Check sheet for the modelled part. Datum: model origin and axes. Units: mm. A direction names the side the tool comes from. Coordinates: 2 decimals unless noted, no trailing zeros. Loops run counter-clockwise (first coordinate to the right, second up) from the corner with the lowest first, then second, coordinate; pieces in that order, holes last. Notation, with made-up numbers: (77.25, 67.25) -> (125.25, 67.25) arc R29 ccw to (125.25, 87.25) -> close; hole circle Ø5 at (53.25, 51). An arc over 180 degrees is marked (long way). Use one line per item in the form item = value.
Autodesk Inventor part; units mm, degrees
ref_plane "YZ Plane" through (0, 0, 0) normal (1, 0, 0) x (0, 1, 0)
ref_plane "XZ Plane" through (0, 0, 0) normal (0, 1, 0) x (-1, 0, 0)
ref_plane "XY Plane" through (0, 0, 0) normal (0, 0, 1) x (1, 0, 0)
sketch "Sketch2" plane through (0, 0, 0) normal (0, 1, 0) x (-1, 0, 0)
  arc A0 (-315.9842, -7.0824) -> (-308.3642, -3.3824) centre (-312.1742, -5.2324) ccw
  line L0 (-312.1742, -5.2324) -> (-308.3642, -3.3824) construction
  line L1 (-312.1742, -5.2324) -> (-315.9842, -7.0824) construction
  line L2 (-343.9242, 64.6176) -> (-343.9242, 51.9176)
  line L3 (-343.9242, 64.6176) -> (-343.9242, 53.0352)
  line L4 (-343.9242, 64.6176) -> (-333.7642, 64.6176)
  arc A1 (-343.9242, 51.9176) -> (-343.2864, 49.1439) centre (-337.5742, 51.9176) ccw
  line L5 (-315.9842, -7.0824) -> (-343.2864, 49.1439)
  line L6 (-333.7642, 64.6176) -> (-333.7642, 50.3868)
  arc A2 (-333.7642, 50.3868) -> (-333.1264, 47.6131) centre (-327.4142, 50.3868) ccw
  line L7 (-333.1264, 47.6131) -> (-308.3642, -3.3824)
  circle A3 centre (-337.5742, 58.2676) radius 2.1463
  circle A4 centre (-312.1742, -5.2324) radius 2.1463
  circle A5 centre (-326.0427, 23.3285) radius 2.1463
  point P0 (0, 0)
  dimension "d0" = 180
  dimension "d1" = 3.81
  dimension "d2" = 10.16
  dimension "d3" = 12.7
  dimension "d4" = 6.35
  dimension "d5" = 31.75
  dimension "d6" = 69.85
  dimension "d7" = 6.35
  dimension "d8" = 4.2926
  dimension "d9" = 4.2926
  dimension "d10" = 6.35
  dimension "d11" = 6.35
  dimension "d12" = 4.2926
  dimension "d13" = 31.75
  dimension "d14" = 4.2354
extrude "Extrusion1" add sketch "Sketch2" along normal blind 1.5875
properties part number "Front Guard"
(1) Tool access check on faces 1 (the flat face through (333.764, 1, 58)), 2 (the flat face through (329, 0, 28)). Record the directions out of +Z, -Z, +X, -X, +Y, -Y that give a thin tool (end or side, any length) a straight path to the whole face; none if there is none.
Established:
face_1 = +Z, -X, +Y, -Y
face_2 = +Z, -Z, +X, -X, -Y
(2) Mould release check, pull along X, two halves, no side actions. Record for faces 3 (the cylindrical face through (339.72, 0.78, 58.17)), 4 (the cylindrical face through (310.24, 0.78, -9)), 5 (the flat face through (320.919, 0.783, 22.472)): +X half, -X half, draft (parallel to the pull), parting line (faces both ways), or undercut.
Established:
face_3 = undercut
face_4 = parting line
face_5 = -X half
(3) Go/stop test with flat-tipped pins: P1, Ø3.5, axis at x = 326.04, z = 23.33, coming from the +Y side; P2, Ø12, axis at x = 325, z = 19.5, coming from the -Y side. Record where each tip stops, or that it passes through.
Established:
P1 = through
P2 = 0
(4) Section check B-B, the plane x = 311. Record the boundary of the cut face in (y, z).
Established:
outline = (0, -9.3) -> (1.59, -9.3) -> (1.59, -7.03) -> (0, -7.03) -> close; (0, -3.44) -> (1.59, -3.44) -> (1.59, 2.05) -> (0, 2.05) -> close
(5) Section check A-A, the plane z = 24. Record the boundary of the cut face in (x, y), plus the area to 3 significant figures.
Established:
outline = (321.66, 0) -> (324, 0) -> (324, 1.59) -> (321.66, 1.59) -> close; (328.08, 0) -> (331.08, 0) -> (331.08, 1.59) -> (328.08, 1.59) -> close
area = 8.48 mm²
(6) Section check C-C, the plane y = 0.25. Record the boundary of the cut face in (x, z).
Established:
outline = (308.36, -3.38) arc R4.24 ccw to (315.98, -7.08) -> (343.29, 49.14) arc R6.35 ccw to (343.92, 51.92) -> (343.92, 64.62) -> (333.76, 64.62) -> (333.76, 50.39) arc R6.35 cw to (333.13, 47.61) -> close; hole circle Ø4.29 at (312.17, -5.23); hole circle Ø4.29 at (326.04, 23.33); hole circle Ø4.29 at (337.57, 58.27)
(7) Scan lines: line 1 along Z through (x, y) = (313, 0.5); line 2 along X through (y, z) = (0.45, 61.5); line 3 along Z through (x, y) = (324.5, 1.1). Record each from-to range of solid material in increasing order.
Established:
line_1 = -9.39 to -7.21, -3.25 to 6.16
line_2 = 333.76 to 343.92
line_3 = 10.46 to 21.84, 24.82 to 29.85
(8) Section check D-D, the plane x = 331.5. Record the boundary of the cut face in (y, z), plus the area to 3 significant figures.
Established:
outline = (0, 24.87) -> (1.59, 24.87) -> (1.59, 44.26) -> (0, 44.26) -> close
area = 30.8 mm²
